The model under review builds one solid part; all positions refer to its coordinate system, in mm. A direction names the side the tool comes from. Coordinates: 2 decimals unless noted, no trailing zeros. Order: outer loops, then holes, each group sorted by start corner. A loop starts at its lowest first (then second) coordinate and runs counter-clockwise, first axis right, second up. Notation, with made-up numbers: (18, 65.5) -> (53, 65.5) arc R24 cw to (53, 102.5) -> close; hole circle Ø11 at (-38.5, 82). An arc over 180 degrees is marked (long way). Use CSV: the item, a comma, the result in double quotes. Start each with the question number.
```python
from build123d import *

# Parameters (mm, degrees)
F0_W      = 110
F0_H      = 110
F1_DEPTH  = 2
F2_W      = 110
F2_H      = 110
F3_DEPTH  = 25
F4_W      = 5
F4_H      = 5
F5_DEPTH  = 23
F6_R      = 1.5
F7_DEPTH  = 10
F8_W      = 15
F8_H      = 114
F9_DEPTH  = 2
F10_R     = 1.5
F11_DEPTH = 2.001
F12_W     = 30
F12_H     = 2
F13_DEPTH = 23
F14_R     = 2
F15_DEPTH = 2.001


with BuildPart() as f1:
    # F0 (on Front) → F1 (new body)
    with BuildSketch(Plane.XZ):
        Rectangle(F0_W, F0_H)
    extrude(amount=F1_DEPTH)

    # F2 (on Front) → F3 (join)
    with BuildSketch(Plane.XZ):
        Polygon((57, 57), (55, 57), (-55, 57), (-57, 57), (-57, 55), (-57, -55), (-57, -57), (-55, -57), (55, -57), (57, -57), (57, -55), (57, 55), align=None)
        Rectangle(F2_W, F2_H, mode=Mode.SUBTRACT)
    extrude(amount=F3_DEPTH)

    # F4 (on face) → F5 (join)
    with BuildSketch(Plane.XZ.offset(2)):
        with Locations((-52.5, 52.5)):
            Rectangle(F4_W, F4_H)
        with Locations((52.5, 52.5)):
            Rectangle(F4_W, F4_H)
        with Locations((-52.5, -52.5)):
            Rectangle(F4_W, F4_H)
        with Locations((52.5, -52.5)):
            Rectangle(F4_W, F4_H)
    extrude(amount=F5_DEPTH)

    # F6 (on face) → F7 (cut)
    with BuildSketch(Plane.XZ.offset(25)):
        with Locations((-53.5, 53.5)):
            Circle(F6_R)
        with Locations((53.5, 53.5)):
            Circle(F6_R)
        with Locations((-53.5, -53.5)):
            Circle(F6_R)
        with Locations((53.5, -53.5)):
            Circle(F6_R)
    extrude(amount=-F7_DEPTH, mode=Mode.SUBTRACT)

    # F8 (on Front) → F9 (join)
    with BuildSketch(Plane.XZ):
        with Locations((-64.5, 0)):
            Rectangle(F8_W, F8_H)
        with Locations((64.5, 0)):
            Rectangle(F8_W, F8_H)
    extrude(amount=F9_DEPTH)

    # F10 (on face) → F11 (cut, through all)
    with BuildSketch(Plane.XZ.offset(2)):
        with Locations((-64.5, 44.430215)):
            Circle(F10_R)
        with Locations((64.5, 44.430215)):
            Circle(F10_R)
        with Locations((-64.5, -44.430215)):
            Circle(F10_R)
        with Locations((64.5, -44.430215)):
            Circle(F10_R)
    extrude(amount=-F11_DEPTH, mode=Mode.SUBTRACT)

    # F12 (on face) → F13 (cut)
    with BuildSketch(Plane.XZ.offset(25)):
        with Locations((0, -56)):
            Rectangle(F12_W, F12_H)
    extrude(amount=-F13_DEPTH, mode=Mode.SUBTRACT)

    # F14 (on face) → F15 (cut, through all)
    with BuildSketch(Plane.XZ.offset(2)):
        with Locations((43.708343, 30)):
            Circle(F14_R)
        with Locations((43.708343, -30)):
            Circle(F14_R)
    extrude(amount=-F15_DEPTH, mode=Mode.SUBTRACT)


solid = f1.part
```
Q1. Add section C-C, the plane x = 33. State the section outline as (y, z) points.
Q2. For faces 4 (the cylindrical face through (65.93, -1.01, 44.88)), 5 (the flat face through (53, -15, -53)), list the 3-axis set-ups (+Z, -Z, +X, -X, +Y, -Y) from which the entire face can be reached by the end or side of a thin tool; tool diameter is ignored.
Q3. Draft analysis for pull direction X (two halves, no side actions). For faces 1 (the flat face through (-33, -13, -55)), 2 (the flat face through (-65, -2, 1)), 3 (the flat face through (-57, -13, 1)), state which applies: +X half, -X half, draft (parallel to the pull), parting line (faces both ways), or undercut.
Q4. Add section A-A, the plane z = 30. State the section outline as (x, y) points, then the cut area to 3 significant figures.
Q5. Add section B-B, the plane x = 64.5. State the section outline as (y, z) points, then the cut area to 3 significant figures.
Q6. Add section D-D, the plane y = -12.75. State the section outline as (x, z) points, then the cut area to 3 significant figures.
Q7. Clearance check with flat-ended pins moving along their axes: pin 1 Ø8 at (y, z) = (-13, 22.5) entering from +X; pin 2 Ø4 at (x, z) = (-64.5, -44.43) entering from -Y; pin 3 Ø1.5 at (x, z) = (53, -53) entering from -Y. State where each tip first meets the part, or that it passes through.
Q8. To check wall thickness, follow probe 1 along X at (y, z) = (-1.75, 44.5); probe 2 along Z at (x, y) = (-53.5, -18); probe 3 along Z at (x, y) = (30, -2.5). State the ranges of each line that lie inside material, in increasing order.
Answer block:
1,outline,"(-25, -57) -> (0, -57) -> (0, 57) -> (-25, 57) -> (-25, 55) -> (-2, 55) -> (-2, -55) -> (-25, -55) -> close"
2,face 4,"+Y, -Y"
2,face 5,"-Y"
3,face 1,"undercut"
3,face 2,"draft"
3,face 3,"-X half"
4,outline,"(-72, -2) -> (-57, -2) -> (-57, -25) -> (-55, -25) -> (-55, -2) -> (41.71, -2) -> (41.71, 0) -> (-72, 0) -> close; (45.71, -2) -> (55, -2) -> (55, -25) -> (57, -25) -> (57, -2) -> (72, -2) -> (72, 0) -> (45.71, 0) -> close"
4,area,"372 mm²"
5,outline,"(-2, -57) -> (0, -57) -> (0, -45.93) -> (-2, -45.93) -> close; (-2, -42.93) -> (0, -42.93) -> (0, 42.93) -> (-2, 42.93) -> close; (-2, 45.93) -> (0, 45.93) -> (0, 57) -> (-2, 57) -> close"
5,area,"216 mm²"
6,outline,"(-57, -57) -> (-15, -57) -> (-15, -55) -> (-50, -55) -> (-50, -50) -> (-55, -50) -> (-55, 50) -> (-50, 50) -> (-50, 55) -> (50, 55) -> (50, 50) -> (55, 50) -> (55, -50) -> (50, -50) -> (50, -55) -> (15, -55) -> (15, -57) -> (57, -57) -> (57, 57) -> (-57, 57) -> close"
6,area,"936 mm²"
7,pin 1,"stops at x = 57"
7,pin 2,"stops at y = -2"
7,pin 3,"stops at y = -15"
8,probe 1,"x = -72 to -66, -63 to 63, 66 to 72"
8,probe 2,"z = -57 to -55, -52 to -50, 50 to 52, 55 to 57"
8,probe 3,"z = -57 to -55, 55 to 57"
